from build123d import *

# Parameters (mm, degrees)
SKETCH2_R   = 15
SKETCH2_R_2 = 10


with BuildPart() as part:
    # Sketch1 → Revolve2 (revolve)
    with BuildSketch(Plane(origin=(0, 0, 0), x_dir=(0, 0, -1), z_dir=(1, 0, 0))):
        with BuildLine():
            Line((0, 30), (-15, 30))
            ThreePointArc((-15, 30), (-107.836049883, 23.108461417), (-200, 10))
            Line((-200, 10), (-200, 0))
            Line((-200, 0), (0, 0))
            Line((0, 0), (0, 30))
        make_face()
    revolve(axis=Axis((0, 30, 0), (0, -1, 0)))

    # Sweep1: sweep along a path in Sketch3
    with BuildLine(Plane.XY) as sweep1_path:
        Line((0, 30), (0, 100))
        ThreePointArc((0, 100), (-8.786796564, 121.213203436), (-30, 130))
        Line((-30, 130), (-200, 130))
    # Sketch2 → Sweep1 (sweep)
    with BuildSketch(Plane(origin=(0, 30, 0), x_dir=(1, 0, 0), z_dir=(0, 1, 0))):
        Circle(SKETCH2_R)
        Circle(SKETCH2_R_2, mode=Mode.SUBTRACT)
    sweep(path=sweep1_path.line)


solid = part.part
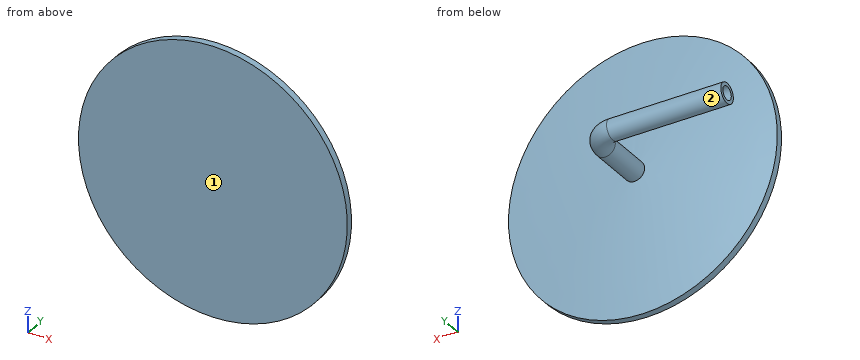
Geometry: final body of the model. Coordinates: model frame, mm. Face numbers are marked on the shaded views. Coordinates: 2 decimals unless noted, no trailing zeros. Order: outer loops, then holes, each group sorted by start corner. A loop starts at its lowest first (then second) coordinate and runs counter-clockwise, first axis right, second up.
(1) Material intervals for probe 1 along X at (y, z) = (83.5, 0); probe 2 along Y at (x, z) = (-99.5, 0), sorted ascending.
(2) Section query B-B (x = -115). State how many separate pieces and enclosed holes the cut face has, plus the area to 3 significant figures.
(3) Section query A-A (y = 46). Return the cut outline in (x, z), plus the area to 3 significant figures.
(4) First-contact query: pin 1 (8 mm diameter, centred on x = -153.5, z = -87, fed in from +Y); pin 2 (5 mm diameter, centred on x = -72.5, z = 93, fed in from +Y); pin 3 (16 mm diameter, centred on x = 4.5, z = 0.5, fed in from +Y). Flat tips, straight axial feed; report the tip coordinate or a pass-through.
(5) Draft query along Y for the marked faces 1 and 2. Return one class per face: pulls with the +Y half, pulls with the -Y half, needs draft (parallel to the pull), parting line crosses it, or undercut.
Solution:
1. probe 1: x = -15 to -10, 10 to 15
1. probe 2: y = 0 to 23.98, 115 to 120, 140 to 145
2. separate pieces: 2
2. enclosed holes: 1
2. area: 6,320 mm2
3. outline: circle Ø30 at (0, 0); hole circle Ø20 at (0, 0)
3. area: 393 mm2
4. pin 1: stops at y = 14.58
4. pin 2: stops at y = 22.27
4. pin 3: stops at y = 136.36
5. face 1: pulls with the -Y half
5. face 2: undercut
